Here's how the part is built. I have some questions about the finished solid (model axes, mm). A direction names the side the tool comes from. Round coordinates to 2 decimals unless told otherwise and drop trailing zeros. Order: outer loops, then holes, each group sorted by start corner. A loop starts at its lowest first (then second) coordinate and runs counter-clockwise, first axis right, second up.
```python
from build123d import *

# Parameters (mm, degrees)
BOSS_EXTRU_1_DEPTH           = 15
ESQUISSE2_W                  = 19
ESQUISSE2_H                  = 23.5
ENL_V_MAT_EXTRU_1_DEPTH      = 12
ESQUISSE6_W                  = 3
ESQUISSE6_H                  = 4.75
ENL_V_MAT_EXTRU_3_DEPTH      = 9
BOSS_EXTRU_2_START           = 33
BOSS_EXTRU_2_DEPTH           = 33
ENL_V_MAT_EXTRU_2_DEPTH      = 12
ESQUISSE7_W                  = 4.75
ESQUISSE7_H                  = 3
ENL_V_MAT_EXTRU_4_DEPTH      = 9
BOSS_EXTRU_3_DEPTH           = 10
ESQUISSE10_W                 = 4.5
ESQUISSE10_H                 = 9
ENL_V_MAT_EXTRU_5_DEPTH      = 10
ESQUISSE11_W                 = 3.5
ESQUISSE11_H                 = 10
ENL_V_MAT_EXTRU_6_DEPTH      = 10
CONG_2_R                     = 2
CONG_3_R                     = 4
CORPS_D_PLACER_COPIER1_ANGLE = 179.5


with BuildPart() as part:
    # Esquisse1 → Boss.-Extru.1 (new body)
    with BuildSketch(Plane(origin=(-30.750548051, -23.495381217, 0), x_dir=(-1, 0, 0), z_dir=(0, 0, -1))):
        with BuildLine():
            Line((-9.363526751, -30.819304804), (-9.363526751, 2.180695196))
            Line((-9.363526751, 2.180695196), (-28.363526751, 2.180695196))
            ThreePointArc((-28.363526751, 2.180695196), (-31.191953876, 1.009122321), (-32.363526751, -1.819304804))
            Line((-32.363526751, -1.819304804), (-32.363526751, -26.819304804))
            ThreePointArc((-32.363526751, -26.819304804), (-31.191953876, -29.647731929), (-28.363526751, -30.819304804))
            Line((-28.363526751, -30.819304804), (-9.363526751, -30.819304804))
        make_face()
    extrude(amount=BOSS_EXTRU_1_DEPTH)

    # Esquisse2 → Enlèv. mat.-Extru.1 (cut)
    with BuildSketch(Plane(origin=(0, 0, -15), x_dir=(-1, 0, 0), z_dir=(0, 0, -1))):
        with Locations((11.8870213, -37.814686021)):
            Rectangle(ESQUISSE2_W, ESQUISSE2_H)
    extrude(amount=-ENL_V_MAT_EXTRU_1_DEPTH, mode=Mode.SUBTRACT)

    # Esquisse6 → Enlèv. mat.-Extru.3 (cut)
    with BuildSketch(Plane(origin=(0, 0, -15), x_dir=(-1, 0, 0), z_dir=(0, 0, -1))):
        with Locations((6.8870213, -23.689686021)):
            Rectangle(ESQUISSE6_W, ESQUISSE6_H)
    extrude(amount=-ENL_V_MAT_EXTRU_3_DEPTH, mode=Mode.SUBTRACT)

    # Esquisse4 → Boss.-Extru.2 (add)
    with BuildSketch(Plane.XY.offset(BOSS_EXTRU_2_START)):
        with BuildLine():
            Line((-21.3870213, -54.314686021), (-21.3870213, -21.314686021))
            Line((-21.3870213, -21.314686021), (-2.3870213, -21.314686021))
            ThreePointArc((-2.3870213, -21.314686021), (0.441405825, -22.486258896), (1.6129787, -25.314686021))
            Line((1.6129787, -25.314686021), (1.6129787, -50.314686021))
            ThreePointArc((1.6129787, -50.314686021), (0.441405825, -53.143113146), (-2.3870213, -54.314686021))
            Line((-2.3870213, -54.314686021), (-21.3870213, -54.314686021))
        make_face()
    extrude(amount=-BOSS_EXTRU_2_DEPTH)

    # Esquisse5 → Enlèv. mat.-Extru.2 (cut)
    with BuildSketch(Plane.ZY.offset(21.3870213)):
        Polygon((0, -44.314686021), (4.75, -44.314686021), (4.75, -25.314686021), (28.25, -25.314686021), (28.25, -44.314686021), (33, -44.314686021), (33, -54.314686021), (0, -54.314686021), align=None)
    extrude(amount=-ENL_V_MAT_EXTRU_2_DEPTH, mode=Mode.SUBTRACT)

    # Esquisse7 → Enlèv. mat.-Extru.4 (cut)
    with BuildSketch(Plane.ZY.offset(21.3870213)):
        with Locations((2.375, -29.814686021)):
            Rectangle(ESQUISSE7_W, ESQUISSE7_H)
    extrude(amount=-ENL_V_MAT_EXTRU_4_DEPTH, mode=Mode.SUBTRACT)

    # Esquisse9 → Boss.-Extru.3 (add)
    with BuildSketch(Plane.ZY.offset(21.3870213)):
        Polygon((28.25, -44.314686021), (33, -44.314686021), (33, -21.314686021), (-3, -21.314686021), (-3, -54.314686021), (0, -54.314686021), (0, -25.314686021), (28.25, -25.314686021), align=None)
    extrude(amount=BOSS_EXTRU_3_DEPTH)

    # Esquisse10 → Enlèv. mat.-Extru.5 (cut)
    with BuildSketch(Plane.XY.offset(33)):
        with Locations((-24.1370213, -31.814686021)):
            Rectangle(ESQUISSE10_W, ESQUISSE10_H)
    extrude(amount=-ENL_V_MAT_EXTRU_5_DEPTH, mode=Mode.SUBTRACT)

    # Esquisse11 → Enlèv. mat.-Extru.6 (cut)
    with BuildSketch(Plane(origin=(0, 0, -3), x_dir=(-1, 0, 0), z_dir=(0, 0, -1))):
        with Locations((26.6370213, -26.314686021)):
            Rectangle(ESQUISSE11_W, ESQUISSE11_H)
    extrude(amount=-ENL_V_MAT_EXTRU_6_DEPTH, mode=Mode.SUBTRACT)

    # Congé2
    cong_2_edges = [part.edges().sort_by_distance(p)[0] for p in [
        (-14.8870213, -21.314686021, -15),
        (0.441405825, -22.486258896, -15),
        (1.6129787, -37.814686021, -15),
        (0.441405825, -53.143113146, -15),
        (-3.8870213, -21.314686021, -15),
        (-11.8870213, -54.314686021, -15),
    ]]
    fillet(cong_2_edges, radius=CONG_2_R)

    # Congé3
    cong_3_edges = [part.edges().sort_by_distance(p)[0] for p in [
        (-31.3870213, -21.314686021, 15),
        (-31.3870213, -54.314686021, -1.5),
        (1.6129787, -37.814686021, 33),
        (-16.8870213, -21.314686021, 33),
        (-5.8870213, -54.314686021, 33),
        (-31.3870213, -32.814686021, 33),
        (0.441405825, -53.143113146, 33),
        (0.441405825, -22.486258896, 33),
    ]]
    fillet(cong_3_edges, radius=CONG_3_R - 0.0001)  # a hair under: the kernel refuses the full size


with BuildPart() as part_1:
    # Corps-Déplacer/Copier1: moved
    add(part.part.rotate(Axis((-14.8870213, -37.814686021, 0), (0, 0, 1)), CORPS_D_PLACER_COPIER1_ANGLE))


solid = part_1.part
```
1. If we section it at C-C, the plane y = -45: State how many separate pieces and enclosed holes the cut face has, and give its area (3 significant figures).
Evaluation:
separate pieces: 3
enclosed holes: 0
area: 589 mm2
2. If we section it at A-A, the plane z = -9: Write out the boundary of the cut face in (x, y), and give its area (3 significant figures).
Evaluation:
outline: (-31.5, -50.17) arc R4 ccw to (-27.53, -54.2) - (-24.53, -54.23) - (-24.49, -49.48) - (-27.49, -49.46) - (-27.28, -25.96) - (-8.28, -26.12) - (-8.24, -21.37) - (-27.24, -21.21) arc R4 ccw to (-31.28, -25.17) - close; (-21.53, -54.26) - (-8.53, -54.37) - (-8.49, -49.62) - (-21.49, -49.51) - close
area: 291 mm2
3. I need wall thicknesses on probe 1 along Z at (x, y) = (-19.5, -36.5); probe 2 along Z at (x, y) = (-3, -41.5); probe 3 along X at (y, z) = (-51.5, -11.5). Which ranges of each line are inside material? Lowest first, please.
Evaluation:
probe 1: z = -3 to 4.75, 28.25 to 33
probe 2: z = -3 to 0, 28.25 to 33
probe 3: x = -31.28 to -24.51, -21.51 to -8.51
4. I'm going to push flat-ended pins straight in: P1, Ø12, axis at y = -27.5, z = 15, coming from the +X side; P2, Ø6, axis at y = -26, z = 4, coming from the +X side; P3, Ø5, axis at x = -21.5, y = -40, coming from the -Z side. Where does each tip first touch, or does it pass through?
Evaluation:
P1: stops at x = -20.24
P2: stops at x = -20.26
P3: stops at z = -3
5. On a 3-axis mill with a long thin cutter (end or side, diameter ignored), from which of +Z, -Z, +X, -X, +Y, -Y can I reach the whole of each face in a straight line? I mean faces 1 (the cylindrical face through (-17.61, -21.86, -14.4)), 2 (the cylindrical face through (-26.047, -53.648, -14.399)), 3 (the cylindrical face through (-30.815, -37.501, -14.399)), 4 (the cylindrical face through (-15.2, -53.11, 31.86)). Say none if no direction works.
Evaluation:
face 1: -Z, +X, +Y
face 2: -Z, -X, -Y
face 3: -Z, -X, +Y
face 4: +Z, -X, -Y
